Read the model definition and answer for the solid it produces. Units are mm, in the model's axes. Give positions to 0.01 mm unless a question says otherwise; leave off trailing zeros. Write each loop counter-clockwise with the first axis right and the second up, starting at its lowest first coordinate (ties: lowest second). Pieces come first, ordered by that corner, then holes.
```python
from build123d import *

# Parameters (mm, degrees)
F0_W     = 94.6727246046
F0_H     = 79.2018212378
F1_DEPTH = 12.7
F2_DEPTH = 25.4
F3_R     = 19.041251915
F3_R_2   = 9.1084784232
F4_DEPTH = 25.4
F5_DEPTH = 38.101


with BuildPart() as f1:
    # F0 (on Front) → F1 (new body)
    with BuildSketch(Plane.XZ):
        with Locations((0, -12.2381839901)):
            Rectangle(F0_W, F0_H)
    extrude(amount=F1_DEPTH)

    # F2 (add): a face of the model
    f2_faces = [f1.faces().sort_by_distance(p)[0] for p in [
        (0, -12.7, -12.2381839901),
    ]]
    extrude(f2_faces, amount=F2_DEPTH)

    # F3 (on face) → F4 (join)
    with BuildSketch(Plane.XZ.offset(38.1)):
        with Locations((0, -10.2754551917)):
            Circle(F3_R)
        with Locations((0, -10.2754551917)):
            Circle(F3_R_2, mode=Mode.SUBTRACT)
    extrude(amount=F4_DEPTH)

    # F5 (cut, through all): a face of the model
    f5_faces = [f1.faces().sort_by_distance(p)[0] for p in [
        (0, -38.1, -10.2754551917),
    ]]
    extrude(f5_faces, amount=-F5_DEPTH, mode=Mode.SUBTRACT)


solid = f1.part
```
Item 1: Find the intervals of material crossed by line 1 along Z through (x, y) = (0, -24); line 2 along Z through (x, y) = (0, -42.75); line 3 along Y through (x, z) = (-6, 21), in increasing order.
Result set:
line 1: z = -51.84 to -19.38, -1.17 to 27.36
line 2: z = -29.32 to -19.38, -1.17 to 8.77
line 3: y = -38.1 to 0
Item 2: Section C-C (y = -6.5) is taken. Write down the section's boundary in (x, z).
Result set:
outline: (-47.34, -51.84) - (47.34, -51.84) - (47.34, 27.36) - (-47.34, 27.36) - close; hole circle Ø18.22 at (0, -10.28)
Item 3: Section B-B (z = -14) is taken. Write down the section's boundary in (x, y), and give its area (3 significant figures).
Result set:
outline: (-47.34, -38.1) - (-18.67, -38.1) - (-18.67, -63.5) - (-8.31, -63.5) - (-8.31, 0) - (-47.34, 0) - close; (8.31, -63.5) - (18.67, -63.5) - (18.67, -38.1) - (47.34, -38.1) - (47.34, 0) - (8.31, 0) - close
area: 3,500 mm2
Item 4: Determine the mould class of faces 1 (the flat face through (-1, 0, -20)), 2 (the cylindrical face through (18.162, -50.622, -4.556)), 3 (the flat face through (-11, -38.1, -29)) for opening direction Y: pulls with the +Y half, pulls with the -Y half, needs draft (parallel to the pull), parting line crosses it, or undercut.
Result set:
face 1: pulls with the +Y half
face 2: needs draft
face 3: pulls with the -Y half
Item 5: Section A-A (x = 0) is taken. Write down the section's boundary in (y, z).
Result set:
outline: (-63.5, -29.32) - (-38.1, -29.32) - (-38.1, -51.84) - (0, -51.84) - (0, -19.38) - (-63.5, -19.38) - close; (-63.5, -1.17) - (0, -1.17) - (0, 27.36) - (-38.1, 27.36) - (-38.1, 8.77) - (-63.5, 8.77) - close
Item 6: Each of these flat-tipped pins is pushed along its axis until it touches: pin 1 Ø10 at (y, z) = (-53, -30) entering from -X; pin 2 Ø4 at (x, z) = (33, -30) entering from -Y; pin 3 Ø8 at (x, y) = (-16.5, -46) entering from +Z; pin 4 Ø16.5 at (x, z) = (0, -10.28) entering from -Y. Where does it stop, or does it pass through?
Result set:
pin 1: stops at x = -12.07
pin 2: stops at y = -38.1
pin 3: stops at z = 4.09
pin 4: passes through
Item 7: Section D-D (z = -26.5) is taken. Write down the section's boundary in (x, y), and give its area (3 significant figures).
Result set:
outline: (-47.34, -38.1) - (-9.97, -38.1) - (-9.97, -63.5) - (9.97, -63.5) - (9.97, -38.1) - (47.34, -38.1) - (47.34, 0) - (-47.34, 0) - close
area: 4,110 mm2
